Part model, mm, in its own coordinate system. Give positions to 0.01 mm unless a question says otherwise; leave off trailing zeros. Order: outer loops, then holes, each group sorted by start corner. A loop starts at its lowest first (then second) coordinate and runs counter-clockwise, first axis right, second up. Notation, with made-up numbers: M 68.5,-15.75 L 87.5,-15.75 A34 ccw 87.5,18.25 Z; hole C 55.25,22 d6. An arc over 180 degrees is marked long. Answer as a JSON object with one key per item and string values.
from build123d import *

# Parameters (mm, degrees)
ESBO_O1_W                = 260
ESBO_O1_H                = 200
ESBO_O1_R                = 12.7
ESBO_O1_R_2              = 30
RESSALTO_EXTRUS_O1_DEPTH = 4.7625


with BuildPart() as part:
    # Esboço1 → Ressalto-extrusão1 (new body)
    with BuildSketch(Plane.XY):
        with Locations((-100, 70)):
            Rectangle(ESBO_O1_W, ESBO_O1_H)
        with Locations(Location((0, 0, 0), (0, 0, 180))):
            Circle(ESBO_O1_R, mode=Mode.SUBTRACT)
        with Locations(Location((-100, 0, 0), (0, 0, 180))):
            Circle(ESBO_O1_R, mode=Mode.SUBTRACT)
        with Locations(Location((-200, 0, 0), (0, 0, 180))):
            Circle(ESBO_O1_R, mode=Mode.SUBTRACT)
        with Locations(Location((-200, 140, 0), (0, 0, 180))):
            Circle(ESBO_O1_R, mode=Mode.SUBTRACT)
        with Locations(Location((-100, 140, 0), (0, 0, 180))):
            Circle(ESBO_O1_R, mode=Mode.SUBTRACT)
        with Locations(Location((0, 140, 0), (0, 0, 180))):
            Circle(ESBO_O1_R, mode=Mode.SUBTRACT)
        with Locations(Location((-100, 70, 0), (0, 0, 180))):
            Circle(ESBO_O1_R_2, mode=Mode.SUBTRACT)
        with Locations(Location((-20, 70, 0), (0, 0, 180))):
            Circle(ESBO_O1_R_2, mode=Mode.SUBTRACT)
        with Locations(Location((-180, 70, 0), (0, 0, 180))):
            Circle(ESBO_O1_R_2, mode=Mode.SUBTRACT)
    extrude(amount=RESSALTO_EXTRUS_O1_DEPTH)


solid = part.part
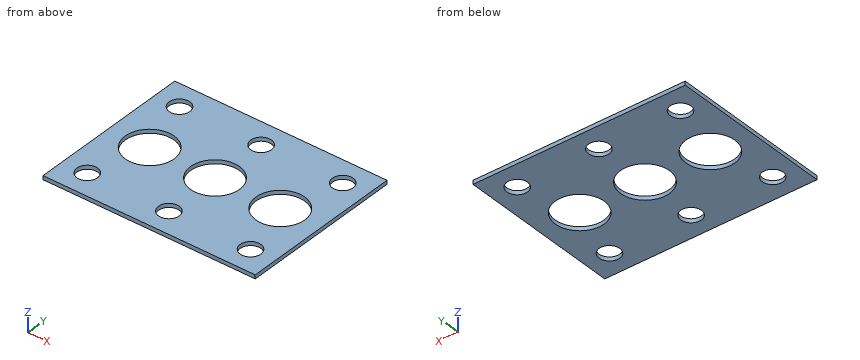
1. Cut at D-D on x = -178. Give the cut face in (y, z), plus the area to 3 significant figures.
Worked answers:
{"outline": "M -30,0 L 40.07,0 L 40.07,4.76 L -30,4.76 Z; M 99.93,0 L 170,0 L 170,4.76 L 99.93,4.76 Z", "area": "667 mm^2"}
2. Cut at C-C on x = -100. Give the cut face in (y, z).
Worked answers:
{"outline": "M -30,0 L -12.7,0 L -12.7,4.76 L -30,4.76 Z; M 12.7,0 L 40,0 L 40,4.76 L 12.7,4.76 Z; M 100,0 L 127.3,0 L 127.3,4.76 L 100,4.76 Z; M 152.7,0 L 170,0 L 170,4.76 L 152.7,4.76 Z"}
3. Pin check, flat tip, straight feed: P1, Ø12, axis at x = -52, y = 127, coming from the -Z side. Stop position of the tip, or through.
Worked answers:
{"P1": "stops at z = 0"}
4. Probe line 1 along Y through (x, z) = (-100, 3.05); line 2 along X through (y, z) = (140, 1.95); line 3 along Y through (x, z) = (-180, 2.75). List the from-to ranges inside material, lowest first.
Worked answers:
{"line 1": "y = -30 to -12.7, 12.7 to 40, 100 to 127.3, 152.7 to 170", "line 2": "x = -230 to -212.7, -187.3 to -112.7, -87.3 to -12.7, 12.7 to 30", "line 3": "y = -30 to 40, 100 to 170"}
5. Cut at B-B on z = 3.6. State how many separate pieces and enclosed holes the cut face has, plus the area to 3 significant figures.
Worked answers:
{"separate pieces": "1", "enclosed holes": "9", "area": "40,500 mm^2"}
6. Cut at A-A on y = 140. Give the cut face in (x, z).
Worked answers:
{"outline": "M -230,0 L -212.7,0 L -212.7,4.76 L -230,4.76 Z; M -187.3,0 L -112.7,0 L -112.7,4.76 L -187.3,4.76 Z; M -87.3,0 L -12.7,0 L -12.7,4.76 L -87.3,4.76 Z; M 12.7,0 L 30,0 L 30,4.76 L 12.7,4.76 Z"}
